Autodesk Inventor part; units mm, degrees
ref_plane "YZ Plane" through (0, 0, 0) normal (1, 0, 0) x (0, 1, 0)
ref_plane "XZ Plane" through (0, 0, 0) normal (0, 1, 0) x (-1, 0, 0)
ref_plane "XY Plane" through (0, 0, 0) normal (0, 0, 1) x (1, 0, 0)
sketch "Sketch1" plane through (0, 0, 0) normal (0, 0, 1) x (1, 0, 0)
  circle A0 centre (0, 0) radius 3.175
  dimension "d0" = 6.35
extrude "Extrusion1" add sketch "Sketch1" along normal mid plane 152.4
sketch "Sketch2" plane through (0, 0, 76.2) normal (0, 0, 1) x (1, 0, 0)
  circle A0 centre (0, 0) radius 3.175
  line L0 (-1.508, 2.794) -> (-1.508, -2.794)
  line L1 (1.508, 2.794) -> (1.508, -2.794)
  line L2 (1.508, -2.794) -> (-1.508, -2.794)
  line L3 (-1.508, 2.794) -> (1.508, 2.794)
  dimension "d3" = 5.588
extrude "Extrusion2" add sketch "Sketch2" along normal blind 6.35 contours L1 L2 L0 L3
sketch "Sketch3" plane through (1.508, -2.794, 76.2) normal (1, 0, 0) x (0, 0, -1)
  line L0 (-6.35, 5.588) -> (-6.35, 0)
  line L1 (0, 0) -> (-6.35, 0)
  line L2 (0, 5.588) -> (0, 0)
  line L3 (0, 5.588) -> (-6.35, 5.588)
  arc A0 (-3.556, 5.588) -> (-3.556, 0) centre (-3.556, 2.794) ccw
  point P0 (76.2, 2.794)
extrude "Extrusion3" cut sketch "Sketch3" against normal blind 6.35 contours L3 A0 L0 | A0 L1 L0
properties part number "piston core"
Part model, mm, in its own coordinate system. A direction names the side the tool comes from. Round coordinates to 2 decimals unless told otherwise and drop trailing zeros. Loops run counter-clockwise (first coordinate to the right, second up) from the corner with the lowest first, then second, coordinate; pieces in that order, holes last. Notation, with made-up numbers: (-4.75, 76) - (33.25, 76) arc R14 cw to (33.25, 100) - close; hole circle Ø7 at (45.5, -25.75). An arc over 180 degrees is marked (long way). Answer as a JSON object with one key per item and string values.
Item 1: Wall check: L1, parallel to Z at x = 2, y = -2.25; L2, parallel to Y at x = 0.25, z = 39.5; L3, parallel to X at y = -1.5, z = -4.5. Give the ranges that are in metal, low to high.
Output:
{"L1": "-76.2 to 76.2", "L2": "-3.17 to 3.17", "L3": "-2.8 to 2.8"}
Item 2: Band-saw the part on C-C on z = 2.5. List the corners of the cut face in (x, y) (3 decimals), plus the area to 3 significant figures.
Output:
{"outline": "circle Ø6.35 at (0, 0)", "area": "31.7 mm2"}
Item 3: Band-saw the part on A-A on y = 0. List the corners of the cut face in (x, z) (3 decimals), plus the area to 3 significant figures.
Output:
{"outline": "(-3.175, -76.2) - (3.175, -76.2) - (3.175, 76.2) - (1.508, 76.2) - (1.508, 82.55) - (-1.508, 82.55) - (-1.508, 76.2) - (-3.175, 76.2) - close", "area": "987 mm2"}
Item 4: Band-saw the part on B-B on x = 0.5. List the corners of the cut face in (y, z), plus the area to 3 significant figures.
Output:
{"outline": "(-3.14, -76.2) - (3.14, -76.2) - (3.14, 76.2) - (2.79, 76.2) - (2.79, 79.76) arc R2.79 ccw to (-2.79, 79.76) - (-2.79, 76.2) - (-3.14, 76.2) - close", "area": "988 mm2"}
Item 5: Tool access for faces 1 (the face through (-1.508, 0, 79)), 2 (the face through (1.508, 0, 79)), 3 (the face through (0, -2.794, 78)), 4 (the face through (0, 2.794, 78)): list every direction of +Z, -Z, +X, -X, +Y, -Y with a clear straight run to the whole face (end or side of a thin tool).
Output:
{"face 1": "+Z, -X, +Y, -Y", "face 2": "+Z, +X, +Y, -Y", "face 3": "+Z, +X, -X, -Y", "face 4": "+Z, +X, -X, +Y"}
Item 6: Pin check, flat tips, straight feed: pin 1 (3 mm diameter, centred on y = 0, z = 80, fed in from -X); pin 2 (2 mm diameter, centred on x = -1.5, z = -27, fed in from +Y); pin 3 (1.8 mm diameter, centred on x = 2.5, y = -0.5, fed in from +Z). Stop position of each tip, or through.
Output:
{"pin 1": "x = -1.51", "pin 2": "y = 3.14", "pin 3": "z = 76.2"}
